Part model, mm, in its own coordinate system. A direction names the side the tool comes from. Round coordinates to 2 decimals unless told otherwise and drop trailing zeros. Loops run counter-clockwise (first coordinate to the right, second up) from the corner with the lowest first, then second, coordinate; pieces in that order, holes last.
1) Band-saw the part on D-D, the plane x = 1. Write the cut outline in (y, z).
2) Band-saw the part on C-C, the plane z = 14. Write the cut outline in (x, y), then the cut area to 3 significant figures.
3) Band-saw the part on A-A, the plane z = 4. Write the cut outline in (x, y), then the cut area to 3 significant figures.
4) Probe line 1 (X direction, y = 0, z = 4); line 2 (Z direction, x = -2.25, y = 0.75); line 3 (Y direction, x = 0.35, z = 3.5). List the from-to ranges inside material, lowest first.
5) Mould opens along Y. For faces 4 (the flat face through (-1.3, -1.4, 0)), 5 (the flat face through (0, 0, 6)), 6 (the flat face through (1.36, -2.39, 12.32)) say: +Y half, -Y half, draft (parallel to the pull), parting line (faces both ways), or undercut.
6) Band-saw the part on B-B, the plane y = 0. Write the cut outline in (x, z).
7) Drop a flat-ended pin along its axis: P1, Ø1, axis at x = 2, z = 13.5, coming from the -Y side. Give the stop position or say it passes through.
8) 3-axis set-ups, long thin cutter, end or side, ignore diameter. For faces 1 (the flat face through (-1.36, 2.39, 12.32)), 2 (the cylindrical face through (-1.5, -0.07, 2.96)), 3 (the cylindrical face through (-1.5, 0.07, 27.96)): which of +Z, -Z, +X, -X, +Y, -Y reach the whole face in a straight line?
from build123d import *

# Parameters (mm, degrees)
F1_DEPTH = 25
F2_R     = 1.5
F3_DEPTH = 6
F4_R     = 1.5
F5_DEPTH = 6


with BuildPart() as f1:
    # F0 (on Top) → F1 (new body)
    with BuildSketch(Plane.XY):
        Polygon((0, 3.1754264805), (-2.75, 1.5877132403), (-2.75, -1.5877132403), (0, -3.1754264805), (2.75, -1.5877132403), (2.75, 1.5877132403), align=None)
    extrude(amount=F1_DEPTH)

    # F2 (on face) → F3 (join)
    with BuildSketch(Plane.XY.offset(25)):
        Circle(F2_R)
    extrude(amount=F3_DEPTH)

    # F4 (on face) → F5 (cut)
    with BuildSketch(Plane(origin=(0, 0, 0), x_dir=(1, 0, 0), z_dir=(0, 0, -1))):
        Circle(F4_R)
    extrude(amount=-F5_DEPTH, mode=Mode.SUBTRACT)


solid = f1.part
Reported:
1. outline: (-2.6, 0) - (-1.12, 0) - (-1.12, 6) - (1.12, 6) - (1.12, 0) - (2.6, 0) - (2.6, 25) - (1.12, 25) - (1.12, 31) - (-1.12, 31) - (-1.12, 25) - (-2.6, 25) - close
2. outline: (-2.75, -1.59) - (0, -3.18) - (2.75, -1.59) - (2.75, 1.59) - (0, 3.18) - (-2.75, 1.59) - close
2. area: 26.2 mm2
3. outline: (-2.75, -1.59) - (0, -3.18) - (2.75, -1.59) - (2.75, 1.59) - (0, 3.18) - (-2.75, 1.59) - close; hole circle Ø3 at (0, 0)
3. area: 19.1 mm2
4. line 1: x = -2.75 to -1.5, 1.5 to 2.75
4. line 2: z = 0 to 25
4. line 3: y = -2.97 to -1.46, 1.46 to 2.97
5. face 4: draft
5. face 5: undercut
5. face 6: -Y half
6. outline: (-2.75, 0) - (-1.5, 0) - (-1.5, 6) - (1.5, 6) - (1.5, 0) - (2.75, 0) - (2.75, 25) - (1.5, 25) - (1.5, 31) - (-1.5, 31) - (-1.5, 25) - (-2.75, 25) - close
7. P1: stops at y = -2.31
8. face 1: +Z, -Z, -X, +Y
8. face 2: -Z
8. face 3: +Z
